```python
from build123d import *

# Parameters (mm, degrees)
BOSS_EXTRUDE1_DEPTH = 2.07
SKETCH3_R           = 16.71
SKETCH3_R_2         = 14.5
EXTRUDE_THIN1_DEPTH = 8.67


with BuildPart() as part:
    # Sketch1 → Boss-Extrude1 (new body)
    with BuildSketch(Plane.XY):
        with BuildLine():
            Line((23.2, -19.7), (-23.2, -19.7))
            ThreePointArc((-23.2, -19.7), (-26.028427125, -18.528427125), (-27.2, -15.7))
            Line((-27.2, -15.7), (-27.2, 15.7))
            ThreePointArc((-27.2, 15.7), (-26.028427125, 18.528427125), (-23.2, 19.7))
            Line((-23.2, 19.7), (23.2, 19.7))
            ThreePointArc((23.2, 19.7), (26.028427125, 18.528427125), (27.2, 15.7))
            Line((27.2, 15.7), (27.2, -15.7))
            ThreePointArc((27.2, -15.7), (26.028427125, -18.528427125), (23.2, -19.7))
        make_face()
    extrude(amount=BOSS_EXTRUDE1_DEPTH)

    # Sketch3 → Extrude-Thin1 (add)
    with BuildSketch(Plane.XY):
        with Locations((-6.958808182, 0)):
            Circle(SKETCH3_R)
        with Locations((-6.958808182, 0)):
            Circle(SKETCH3_R_2, mode=Mode.SUBTRACT)
    extrude(amount=EXTRUDE_THIN1_DEPTH)


solid = part.part
```
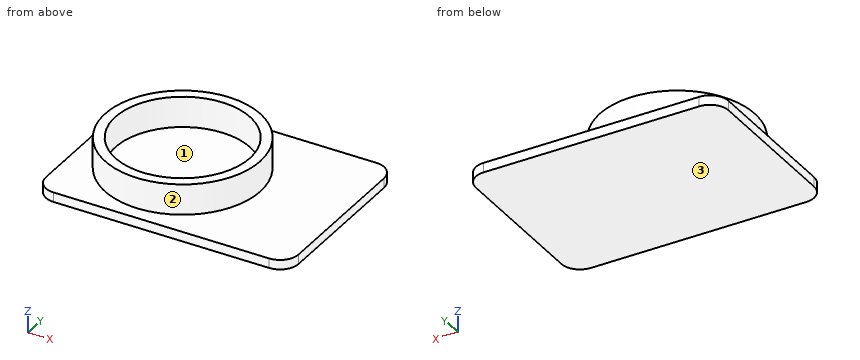
Read the model definition and answer for the solid it produces. Units are mm, in the model's axes. Face numbers are marked on the shaded views. Give positions to 0.01 mm unless a question says otherwise; leave off trailing zeros. Write each loop counter-clockwise with the first axis right and the second up, starting at its lowest first coordinate (ties: lowest second). Pieces come first, ordered by that corner, then holes. Notation, with made-up numbers: (-18.5, 82) -> (-5.5, 82) arc R29 cw to (-5.5, 118) -> close; hole circle Ø7 at (75, 6.5). An arc over 180 degrees is marked (long way). Answer as a JSON object with one key per item and string values.
1) Flat-ended cylindrical pins translate along their axes: pin 1 Ø1 at (x, y) = (9, 3) entering from -Z; pin 2 Ø1 at (x, z) = (-5.5, 4) entering from +Y; pin 3 Ø1.5 at (y, z) = (-14, 3.5) entering from -X; pin 4 Ø8.5 at (x, y) = (0.5, -3) entering from +Z. Find the tip coordinate at first contact, or state that the pin passes through.
Findings below:
{"pin 1": "stops at z = 0", "pin 2": "stops at y = 16.68", "pin 3": "stops at x = -17.14", "pin 4": "stops at z = 2.07"}
2) Section A-A on y = 0 is taken. Write down the section's boundary in (x, z), then the cut area to 3 significant figures.
Findings below:
{"outline": "(-27.2, 0) -> (27.2, 0) -> (27.2, 2.07) -> (9.75, 2.07) -> (9.75, 8.67) -> (7.54, 8.67) -> (7.54, 2.07) -> (-21.46, 2.07) -> (-21.46, 8.67) -> (-23.67, 8.67) -> (-23.67, 2.07) -> (-27.2, 2.07) -> close", "area": "142 mm^2"}
3) Section B-B on z = 5.75 is taken. Write down the section's boundary in (x, y).
Findings below:
{"outline": "circle Ø33.42 at (-6.96, 0); hole circle Ø29 at (-6.96, 0)"}
4) For a pull along Y with two mould halves and no side action, classify the marked faces 1, 2 and 3 as pulls with the +Y half, pulls with the -Y half, needs draft (parallel to the pull), parting line crosses it, or undercut.
Findings below:
{"face 1": "undercut", "face 2": "parting line crosses it", "face 3": "needs draft"}
5) Straight lines are drawn through the part: probe 1 along Y at (x, z) = (-7.5, 7.25); probe 2 along X at (y, z) = (0, 5); probe 3 along Z at (x, y) = (2, 3.5). For each, find the intervals that lie inside material, in ascending order. Write a range as from..to.
Findings below:
{"probe 1": "y = -16.7..-14.49, 14.49..16.7", "probe 2": "x = -23.67..-21.46, 7.54..9.75", "probe 3": "z = 0..2.07"}
6) Section C-C on x = -13 is taken. Write down the section's boundary in (y, z).
Findings below:
{"outline": "(-19.7, 0) -> (19.7, 0) -> (19.7, 2.07) -> (15.58, 2.07) -> (15.58, 8.67) -> (13.18, 8.67) -> (13.18, 2.07) -> (-13.18, 2.07) -> (-13.18, 8.67) -> (-15.58, 8.67) -> (-15.58, 2.07) -> (-19.7, 2.07) -> close"}
